Here's how the part is built. I have some questions about the finished solid (model axes, mm). Round coordinates to 2 decimals unless told otherwise and drop trailing zeros. Write each loop counter-clockwise with the first axis right and the second up, starting at its lowest first coordinate (ties: lowest second). Pieces come first, ordered by that corner, then holes. Notation, with made-up numbers: (39, 55) - (60, 55) arc R32 ccw to (60, 85) - close; hole circle Ø1 at (-34.75, -20). An arc over 180 degrees is marked (long way). One line per item, written item: value. Start each with the question number.
Item 1: Imagine slicing it at D-D, the plane y = 15. Please give me the cut outline in (x, z), then the cut area to 3 significant figures.
Item 2: Imagine slicing it at A-A, the plane x = 47.5. Please give me the cut outline in (y, z), then the cut area to 3 significant figures.
Item 3: Imagine slicing it at B-B, the plane x = 81. Please give me the cut outline in (y, z) (3 decimals), then the cut area to 3 significant figures.
Item 4: For P1, Ø1.6, axis at x = 61.5, y = 8, coming from the -Z side; P2, Ø2.5, axis at x = 60.63, y = 7.08, coming from the -Z side, each with a flat end and sliding along its axis, tell me the tip position at first contact or that it passes through.
Item 5: If I drill on line 1 (X direction, y = 42.5, z = 3.45); line 2 (Y direction, x = 81, z = 1.75) (3 decimals); line 3 (X direction, y = 48, z = 2.9), over which ranges is the centre line in solid material (lowest first)?
Item 6: Imagine slicing it at C-C, the plane z = 1.05. Count the separate pieces of the cut face and the enclosed holes in it, then the cut area to 3 significant figures.
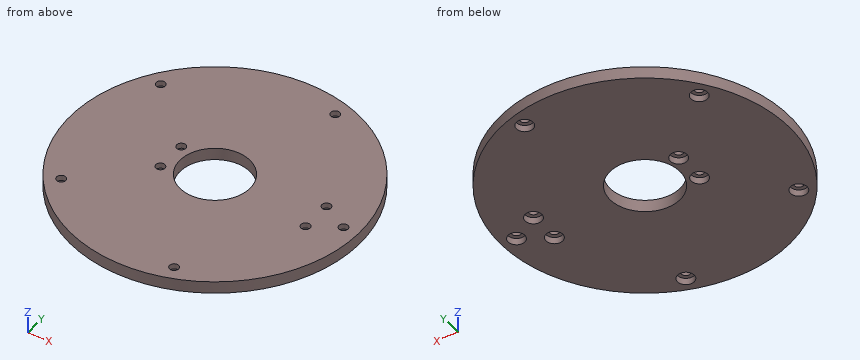
```python
from build123d import *

# Parameters (mm, degrees)
SKETCH1_R           = 47.5
SKETCH1_R_2         = 2.75
SKETCH1_R_3         = 11.5
SKETCH1_R_4         = 1.5
BOSS_EXTRUDE2_DEPTH = 4
SKETCH1_5_R         = 2.75
SKETCH1_5_R_2       = 1.5
CUT_EXTRUDE1_DEPTH  = 2.2


with BuildPart() as part:
    # Sketch1 → Boss-Extrude2 (new body)
    with BuildSketch(Plane.XY):
        with Locations((47.5, 47.5)):
            Circle(SKETCH1_R)
        with Locations((81, 42.125)):
            Circle(SKETCH1_R_2, mode=Mode.SUBTRACT)
        with Locations((90, 47.5)):
            Circle(SKETCH1_R_2, mode=Mode.SUBTRACT)
        with Locations((81, 52.625)):
            Circle(SKETCH1_R_2, mode=Mode.SUBTRACT)
        with Locations((60.633222261, 87.919901943)):
            Circle(SKETCH1_R_2, mode=Mode.SUBTRACT)
        with Locations((13.116777739, 72.480873222)):
            Circle(SKETCH1_R_2, mode=Mode.SUBTRACT)
        with Locations((33, 52.625)):
            Circle(SKETCH1_R_2, mode=Mode.SUBTRACT)
        with Locations((33, 42.125)):
            Circle(SKETCH1_R_2, mode=Mode.SUBTRACT)
        with Locations((60.633222261, 7.080098057)):
            Circle(SKETCH1_R_2, mode=Mode.SUBTRACT)
        with Locations((13.116777739, 22.519126778)):
            Circle(SKETCH1_R_2, mode=Mode.SUBTRACT)
        with Locations((47.5, 47.5)):
            Circle(SKETCH1_R_3, mode=Mode.SUBTRACT)
        with Locations((13.116777739, 72.480873222)):
            Circle(SKETCH1_R_2)
        with Locations((13.116777739, 72.480873222)):
            Circle(SKETCH1_R_4, mode=Mode.SUBTRACT)
        with Locations((60.633222261, 87.919901943)):
            Circle(SKETCH1_R_2)
        with Locations((60.633222261, 87.919901943)):
            Circle(SKETCH1_R_4, mode=Mode.SUBTRACT)
        with Locations((33, 52.625)):
            Circle(SKETCH1_R_2)
        with Locations((33, 52.625)):
            Circle(SKETCH1_R_4, mode=Mode.SUBTRACT)
        with Locations((81, 52.625)):
            Circle(SKETCH1_R_2)
        with Locations((81, 52.625)):
            Circle(SKETCH1_R_4, mode=Mode.SUBTRACT)
        with Locations((90, 47.5)):
            Circle(SKETCH1_R_2)
        with Locations((90, 47.5)):
            Circle(SKETCH1_R_4, mode=Mode.SUBTRACT)
        with Locations((81, 42.125)):
            Circle(SKETCH1_R_2)
        with Locations((81, 42.125)):
            Circle(SKETCH1_R_4, mode=Mode.SUBTRACT)
        with Locations((33, 42.125)):
            Circle(SKETCH1_R_2)
        with Locations((33, 42.125)):
            Circle(SKETCH1_R_4, mode=Mode.SUBTRACT)
        with Locations((13.116777739, 22.519126778)):
            Circle(SKETCH1_R_2)
        with Locations((13.116777739, 22.519126778)):
            Circle(SKETCH1_R_4, mode=Mode.SUBTRACT)
        with Locations((60.633222261, 7.080098057)):
            Circle(SKETCH1_R_2)
        with Locations((60.633222261, 7.080098057)):
            Circle(SKETCH1_R_4, mode=Mode.SUBTRACT)
    extrude(amount=BOSS_EXTRUDE2_DEPTH)

    # Sketch1_5 → Cut-Extrude1 (cut)
    with BuildSketch(Plane.XY):
        with Locations((33, 52.625)):
            Circle(SKETCH1_5_R)
        with Locations((33, 52.625)):
            Circle(SKETCH1_5_R_2, mode=Mode.SUBTRACT)
        with Locations((33, 42.125)):
            Circle(SKETCH1_5_R)
        with Locations((33, 42.125)):
            Circle(SKETCH1_5_R_2, mode=Mode.SUBTRACT)
        with Locations((13.116777739, 22.519126778)):
            Circle(SKETCH1_5_R)
        with Locations((13.116777739, 22.519126778)):
            Circle(SKETCH1_5_R_2, mode=Mode.SUBTRACT)
        with Locations((13.116777739, 72.480873222)):
            Circle(SKETCH1_5_R)
        with Locations((13.116777739, 72.480873222)):
            Circle(SKETCH1_5_R_2, mode=Mode.SUBTRACT)
        with Locations((60.633222261, 87.919901943)):
            Circle(SKETCH1_5_R)
        with Locations((60.633222261, 87.919901943)):
            Circle(SKETCH1_5_R_2, mode=Mode.SUBTRACT)
        with Locations((81, 52.625)):
            Circle(SKETCH1_5_R)
        with Locations((81, 52.625)):
            Circle(SKETCH1_5_R_2, mode=Mode.SUBTRACT)
        with Locations((90, 47.5)):
            Circle(SKETCH1_5_R)
        with Locations((90, 47.5)):
            Circle(SKETCH1_5_R_2, mode=Mode.SUBTRACT)
        with Locations((81, 42.125)):
            Circle(SKETCH1_5_R)
        with Locations((81, 42.125)):
            Circle(SKETCH1_5_R_2, mode=Mode.SUBTRACT)
        with Locations((60.633222261, 7.080098057)):
            Circle(SKETCH1_5_R)
        with Locations((60.633222261, 7.080098057)):
            Circle(SKETCH1_5_R_2, mode=Mode.SUBTRACT)
    extrude(amount=CUT_EXTRUDE1_DEPTH, mode=Mode.SUBTRACT)


solid = part.part
```
Values follow:
1. outline: (12.86, 0) - (82.14, 0) - (82.14, 4) - (12.86, 4) - close
1. area: 277 mm^2
2. outline: (0, 0) - (36, 0) - (36, 4) - (0, 4) - close; (59, 0) - (95, 0) - (95, 4) - (59, 4) - close
2. area: 288 mm^2
3. outline: (13.825, 0) - (39.375, 0) - (39.375, 2.2) - (40.625, 2.2) - (40.625, 4) - (13.825, 4) - close; (43.625, 2.2) - (44.875, 2.2) - (44.875, 0) - (49.875, 0) - (49.875, 2.2) - (51.125, 2.2) - (51.125, 4) - (43.625, 4) - close; (54.125, 2.2) - (55.375, 2.2) - (55.375, 0) - (81.175, 0) - (81.175, 4) - (54.125, 4) - close
3. area: 234 mm^2
4. P1: stops at z = 2.2
4. P2: passes through
5. line 1: x = 0.26 to 31.55, 34.45 to 37.14, 57.86 to 79.55, 82.45 to 94.74
5. line 2: y = 13.825 to 39.375, 44.875 to 49.875, 55.375 to 81.175
5. line 3: x = 0 to 36.01, 58.99 to 88.59, 91.41 to 95
6. separate pieces: 1
6. enclosed holes: 10
6. area: 6,460 mm^2
